The listing builds one solid part. Answer for the finished solid, in the listing's coordinates (mm). Coordinates: 2 decimals unless noted, no trailing zeros. Loops run counter-clockwise (first coordinate to the right, second up) from the corner with the lowest first, then second, coordinate; pieces in that order, holes last. Notation, with made-up numbers: (38.5, 30) - (90.5, 30) arc R19 cw to (90.5, 35) - close; hole circle Ø3 at (-37.75, 57). An arc over 180 degrees is marked (long way). Put each result on its own line as item: value.
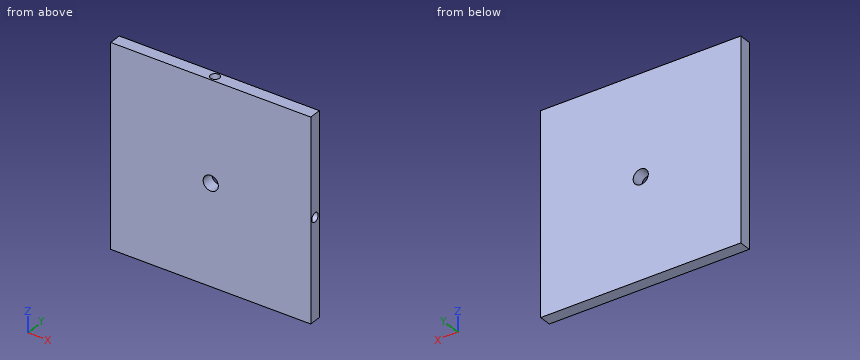
```python
from build123d import *

# Parameters (mm, degrees)
SKETCH1_W                       = 419.1
SKETCH1_H                       = 419.1
SKETCH1_R                       = 15.875
BOSS_EXTRUDE1_DEPTH             = 25.4
F_3_4_0_75_DIAMETER_HOLE2_D     = 19.05
F_3_4_0_75_DIAMETER_HOLE2_DEPTH = 76.2
F_3_4_0_75_DIAMETER_HOLE2_TIP   = 5.723197396
F_3_4_0_75_DIAMETER_HOLE1_D     = 19.05
F_3_4_0_75_DIAMETER_HOLE1_DEPTH = 76.2
F_3_4_0_75_DIAMETER_HOLE1_TIP   = 5.723197396


with BuildPart() as part:
    # Sketch1 → Boss-Extrude1 (new body)
    with BuildSketch(Plane(origin=(0, 0, 0), x_dir=(1, 0, 0), z_dir=(0, 1, 0))):
        Rectangle(SKETCH1_W, SKETCH1_H)
        Circle(SKETCH1_R, mode=Mode.SUBTRACT)
    extrude(amount=BOSS_EXTRUDE1_DEPTH)

    # 3/4 (0.75) Diameter Hole2
    with Locations(Plane(origin=(209.55, 0, 0), x_dir=(0, 0, -1), z_dir=(1, 0, 0))):
        with Locations((0, 12.7)):
            Hole(F_3_4_0_75_DIAMETER_HOLE2_D / 2, depth=F_3_4_0_75_DIAMETER_HOLE2_DEPTH)
            with Locations((0, 0, -(F_3_4_0_75_DIAMETER_HOLE2_DEPTH + F_3_4_0_75_DIAMETER_HOLE2_TIP / 2))):  # 118° drill point
                Cone(0, F_3_4_0_75_DIAMETER_HOLE2_D / 2, F_3_4_0_75_DIAMETER_HOLE2_TIP, mode=Mode.SUBTRACT)

    # 3/4 (0.75) Diameter Hole1
    with Locations(Plane.XY.offset(209.55)):
        with Locations((0, 12.7)):
            Hole(F_3_4_0_75_DIAMETER_HOLE1_D / 2, depth=F_3_4_0_75_DIAMETER_HOLE1_DEPTH)
            with Locations((0, 0, -(F_3_4_0_75_DIAMETER_HOLE1_DEPTH + F_3_4_0_75_DIAMETER_HOLE1_TIP / 2))):  # 118° drill point
                Cone(0, F_3_4_0_75_DIAMETER_HOLE1_D / 2, F_3_4_0_75_DIAMETER_HOLE1_TIP, mode=Mode.SUBTRACT)


solid = part.part
```
1) The part is cut by section A-A (z = 155). Give the vertices of the cut face in (x, y) (3 decimals).
Found:
outline: (-209.55, 0) - (209.55, 0) - (209.55, 25.4) - (-209.55, 25.4) - close; hole circle Ø19.05 at (0, 12.7)
2) This flat-tipped pin is pushed along its axis until it touches: pin 1 (1.5 mm diameter, centred on x = -145.5, z = -131.5, fed in from -Y). Where does it stop, or does it pass through?
Found:
pin 1: stops at y = 0
3) Straight lines are drawn through the part: L1, parallel to Z at x = 149, y = 12.7 (3 decimals); L2, parallel to Y at x = 171, z = 0 (3 decimals); L3, parallel to X at y = 11.5, z = 0 (3 decimals). For each, find the intervals that lie inside material, in ascending order. Write a range as [from, to].
Found:
L1: z = [-209.55, -9.525], [9.525, 209.55]
L2: y = [0, 3.175], [22.225, 25.4]
L3: x = [-209.55, -15.875], [15.875, 128.348]
